Job drawing, mm, ordinate dimensions from the low corner. One solid piece. Round coordinates to 2 decimals unless told otherwise and drop trailing zeros. Order: outer loops, then holes, each group sorted by start corner. A loop starts at its lowest first (then second) coordinate and runs counter-clockwise, first axis right, second up. Notation, with made-up numbers: (16, 80) -> (57, 80) arc R17 cw to (57, 109) -> close; hole circle Ø2 at (-17.5, -39.75). An arc over 180 degrees is marked (long way). Return JSON: item names as keys, results as strings. Group by question number.
Q1. Cut at D-D (x = 22.5). Write the cut outline in (y, z).
Q2. Cut at C-C (y = 17.5). Write the cut outline in (x, z), then the cut area to 3 significant figures.
Q3. Mould opens along X. For the marked faces 1, 2 and 3 say: +X half, -X half, draft (parallel to the pull), parting line (faces both ways), or undercut.
Q4. Cut at B-B (z = 35). Write the cut outline in (x, y).
Q5. Probe line 1 along Z through (x, y) = (20, 37.5); line 2 along X through (y, z) = (39, 40); line 3 along X through (y, z) = (38.5, 29). List the from-to ranges inside material, lowest first.
Q6. Cut at A-A (x = 60). Write the cut outline in (y, z), then the cut area to 3 significant figures.
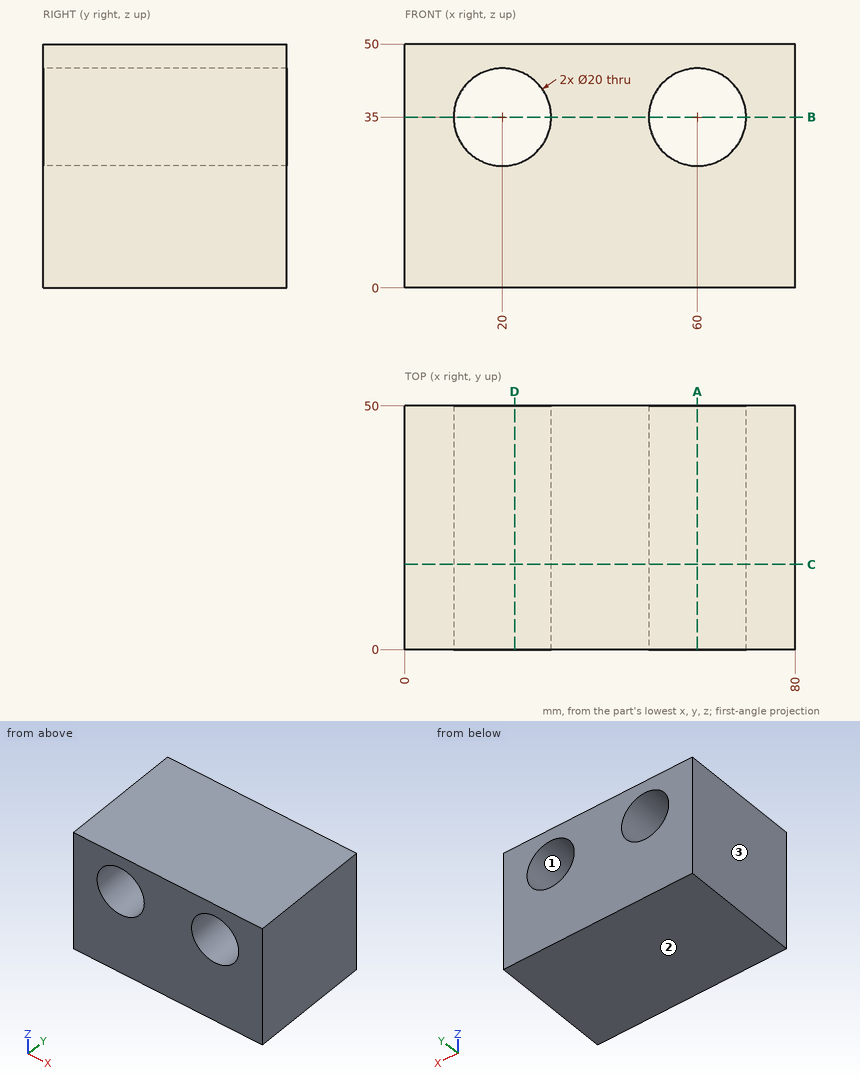
Solution:
{
 "1": {"outline": "(0, 0) -> (50, 0) -> (50, 25.32) -> (0, 25.32) -> close; (0, 44.68) -> (50, 44.68) -> (50, 50) -> (0, 50) -> close"},
 "2": {"outline": "(0, 0) -> (80, 0) -> (80, 50) -> (0, 50) -> close; hole circle Ø20 at (20, 35); hole circle Ø20 at (60, 35)", "area": "3,370 mm²"},
 "3": {"face 1": "undercut", "face 2": "draft", "face 3": "-X half"},
 "4": {"outline": "(0, 0) -> (10, 0) -> (10, 50) -> (0, 50) -> close; (30, 0) -> (50, 0) -> (50, 50) -> (30, 50) -> close; (70, 0) -> (80, 0) -> (80, 50) -> (70, 50) -> close"},
 "5": {"line 1": "z = 0 to 25, 45 to 50", "line 2": "x = 0 to 11.34, 28.66 to 51.34, 68.66 to 80", "line 3": "x = 0 to 12, 28 to 52, 68 to 80"},
 "6": {"outline": "(0, 0) -> (50, 0) -> (50, 25) -> (0, 25) -> close; (0, 45) -> (50, 45) -> (50, 50) -> (0, 50) -> close", "area": "1,500 mm²"}
}
